from build123d import *

# Parameters (mm, degrees)
BACKPLATELEFT_MIRRORED_OUTLINE_R   = 2.1
BACKPLATELEFT_MIRRORED_OUTLINE_R_2 = 10
BACKPLATELEFT_MIRRORED_DEPTH       = 3
SKETCH2_W                          = 40
SKETCH2_H                          = 103.465043027
CUT_EXTRUDE1_DEPTH                 = 10
SKETCH3_W                          = 25.884261779
SKETCH3_H                          = 20.988460011
BOSS_EXTRUDE1_DEPTH                = 3
FILLET1_R                          = 10
CUT_EXTRUDE2_DEPTH                 = 97.379458392
CUT_EXTRUDE2_DEPTH_BACK            = 97.379458392
SKETCH4_W                          = 88
SKETCH4_H                          = 4


# Read off the part's stored shape, not the designer's step: backPlateLeft_Mirrored
with BuildPart() as part:
    # backPlateLeft_Mirrored outline → backPlateLeft_Mirrored (new body)
    with BuildSketch(Plane(origin=(0, 0, 0), x_dir=(1, 0, 0), z_dir=(0, 1, 0))):
        with BuildLine():
            Line((-24, 24), (-24, -39))
            Line((-24, -39), (64, -39))
            Line((64, -39), (64, 135))
            ThreePointArc((64, 135), (62.242640687, 139.242640687), (58, 141))
            Line((58, 141), (30, 141))
            ThreePointArc((30, 141), (25.757359313, 139.242640687), (24, 135))
            Line((24, 135), (24, 72))
            Line((24, 72), (14, 72))
            ThreePointArc((14, 72), (9.757359313, 70.242640687), (8, 66))
            Line((8, 66), (8, 26))
            ThreePointArc((8, 26), (7.414213562, 24.585786438), (6, 24))
            Line((6, 24), (-24, 24))
        make_face()
        with Locations((-16, -16)):
            Circle(BACKPLATELEFT_MIRRORED_OUTLINE_R, mode=Mode.SUBTRACT)
        with Locations((16, -16)):
            Circle(BACKPLATELEFT_MIRRORED_OUTLINE_R, mode=Mode.SUBTRACT)
        with Locations((-16, 16)):
            Circle(BACKPLATELEFT_MIRRORED_OUTLINE_R, mode=Mode.SUBTRACT)
        with Locations((16, 16)):
            Circle(BACKPLATELEFT_MIRRORED_OUTLINE_R, mode=Mode.SUBTRACT)
        with Locations((16, 32)):
            Circle(BACKPLATELEFT_MIRRORED_OUTLINE_R, mode=Mode.SUBTRACT)
        with Locations((44, 0)):
            Circle(BACKPLATELEFT_MIRRORED_OUTLINE_R_2, mode=Mode.SUBTRACT)
        with Locations((44, 35)):
            Circle(BACKPLATELEFT_MIRRORED_OUTLINE_R_2, mode=Mode.SUBTRACT)
        with Locations((16, 64)):
            Circle(BACKPLATELEFT_MIRRORED_OUTLINE_R, mode=Mode.SUBTRACT)
        with Locations((44, 70)):
            Circle(BACKPLATELEFT_MIRRORED_OUTLINE_R_2, mode=Mode.SUBTRACT)
        with Locations((44, 105)):
            Circle(BACKPLATELEFT_MIRRORED_OUTLINE_R_2, mode=Mode.SUBTRACT)
    extrude(amount=BACKPLATELEFT_MIRRORED_DEPTH)

    # Sketch2 → Cut-Extrude1 (cut)
    with BuildSketch(Plane(origin=(0, 3, 0), x_dir=(1, 0, 0), z_dir=(0, 1, 0))):
        with Locations((44, 123.732521514)):
            Rectangle(SKETCH2_W, SKETCH2_H)
    extrude(amount=-CUT_EXTRUDE1_DEPTH, mode=Mode.SUBTRACT)

    # Sketch3 → Boss-Extrude1 (add)
    with BuildSketch(Plane(origin=(0, 3, 0), x_dir=(1, 0, 0), z_dir=(0, 1, 0))):
        with Locations((44.305953134, 61.505769994)):
            Rectangle(SKETCH3_W, SKETCH3_H)
    extrude(amount=-BOSS_EXTRUDE1_DEPTH)

    # Fillet1
    fillet1_edges = [part.edges().sort_by_distance(p)[0] for p in [
        (64, 1.5, -72),
    ]]
    fillet(fillet1_edges, radius=FILLET1_R)

    # Sketch4 → Cut-Extrude2 (cut, two sides: drawn at the far end of the back side and taken through both)
    with BuildSketch(Plane(origin=(0, 3, 0), x_dir=(1, 0, 0), z_dir=(0, 1, 0)).offset(-CUT_EXTRUDE2_DEPTH_BACK)):
        with Locations((20, -37)):
            Rectangle(SKETCH4_W, SKETCH4_H)
    extrude(amount=CUT_EXTRUDE2_DEPTH + CUT_EXTRUDE2_DEPTH_BACK, mode=Mode.SUBTRACT)


solid = part.part
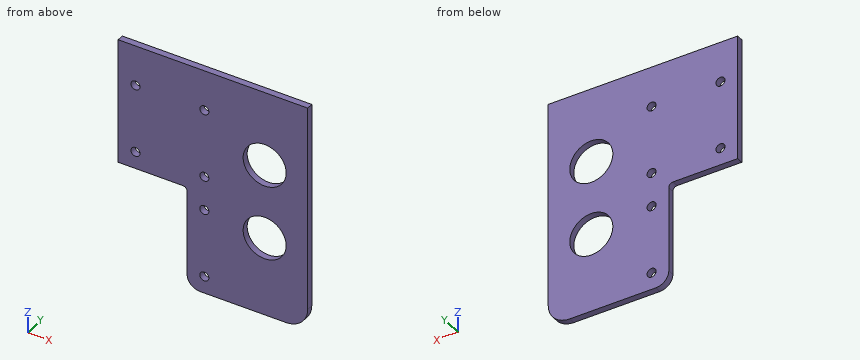
The listing builds one solid part. Answer for the finished solid, in the listing's coordinates (mm). Give positions to 0.01 mm unless a question says otherwise; leave off trailing zeros. Order: outer loops, then holes, each group sorted by start corner. A loop starts at its lowest first (then second) coordinate and runs counter-clockwise, first axis right, second up. Notation, with made-up numbers: (-13, -5.5) -> (-6, -5.5) arc R18 cw to (-6, 26.5) -> close; hole circle Ø4 at (49.25, -13.5). An arc over 180 degrees is marked (long way). Put each result on its own line as item: value.
Item 1: Given P1, Ø16, axis at x = 44, z = 0, coming from the +Y side, flat-ended and moving along its own axis, determine where the tip first touches the part or whether it passes through.
Established:
P1: passes through
Item 2: A cutting plane is placed at A-A on z = 16. Give the vertices of the cut face in (x, y), plus the area to 3 significant figures.
Established:
outline: (-24, 0) -> (-18.1, 0) -> (-18.1, 3) -> (-24, 3) -> close; (-13.9, 0) -> (13.9, 0) -> (13.9, 3) -> (-13.9, 3) -> close; (18.1, 0) -> (64, 0) -> (64, 3) -> (18.1, 3) -> close
area: 239 mm^2
Item 3: A cutting plane is placed at D-D on z = 0. Give the vertices of the cut face in (x, y).
Established:
outline: (-24, 0) -> (34, 0) -> (34, 3) -> (-24, 3) -> close; (54, 0) -> (64, 0) -> (64, 3) -> (54, 3) -> close
Item 4: Straight lines are drawn through the part: line 1 (Z direction, x = 44, y = 0.65); line 2 (Z direction, x = 16, y = 0.75); line 3 (X direction, y = 2.3, z = 16). For each, find the intervals that lie inside material, in ascending order.
Established:
line 1: z = -72 to -45, -25 to -10, 10 to 35
line 2: z = -72 to -66.1, -61.9 to -34.1, -29.9 to -18.1, -13.9 to 13.9, 18.1 to 35
line 3: x = -24 to -18.1, -13.9 to 13.9, 18.1 to 64
Item 5: A cutting plane is placed at B-B on x = -16. Give the vertices of the cut face in (y, z).
Established:
outline: (0, -24) -> (3, -24) -> (3, -18.1) -> (0, -18.1) -> close; (0, -13.9) -> (3, -13.9) -> (3, 13.9) -> (0, 13.9) -> close; (0, 18.1) -> (3, 18.1) -> (3, 35) -> (0, 35) -> close
Item 6: A cutting plane is placed at C-C on y = 1.8. Count the separate pieces of the cut face and the enclosed holes in it, plus the area to 3 significant figures.
Established:
separate pieces: 1
enclosed holes: 8
area: 7,140 mm^2
